Could you check a few things on this model? Use its own coordinates, in mm. A direction names the side the tool comes from. Give positions to 0.01 mm unless a question says otherwise; leave off trailing zeros. Loops run counter-clockwise (first coordinate to the right, second up) from the corner with the lowest first, then second, coordinate; pieces in that order, holes last. Notation, with made-up numbers: (43.5, -21.5) -> (101.5, -21.5) arc R15 cw to (101.5, -3.5) -> close; hole circle Ø5 at (69, 3.5). An arc over 180 degrees is marked (long way). Write each question's results on one line, items separated by ' | '. Start each with the question number.
Q1. Which directions (+Z, -Z, +X, -X, +Y, -Y) give clear straight access to the entire face, cutting with the end or side of a thin tool? Please do faces 5 (the face through (-11.112, 43, 1)), 6 (the face through (30, -30, -50.8)), 7 (the face through (-52.07, 47.74, 0.71)).
Q2. If we section it at D-D, the plane x = 274.5: List the corners of the cut face in (y, z) for me (3 decimals).
Q3. Will these pins go through, and if not, where does the flat tip stop? P1, Ø6, axis at x = 135.5, z = -8, coming from the +Y side; P2, Ø14, axis at y = 44.5, z = -8.5, coming from the +X side; P3, Ø2, axis at x = 180.5, y = -74, coming from the -Z side (3 decimals).
Q4. If we section it at C-C, the plane z = -23.5: List the corners of the cut face in (x, y) for me.
Q5. If I drill on line 1 along Z through (x, y) = (100, -20) (3 decimals); line 2 along X through (y, z) = (8, -6); line 3 along X through (y, z) = (-16, 14), over which ranges is the centre line in solid material (lowest first)?
Q6. If we section it at B-B, the plane x = 0: List the corners of the cut face in (y, z) for me (3 decimals), plus the area to 3 significant figures.
Q7. If we section it at A-A, the plane y = 0: List the corners of the cut face in (x, z) for me (3 decimals).
Q8. We'd pull the mould along Y, two halves only. Please class faces 1 (the face through (136.315, 49.845, 0.222)), 2 (the face through (1.519, -38.095, 0.711)), 3 (the face through (172.854, -100.986, 0.222)), 4 (the face through (30, -30, 50.8)): released by +Y, released by -Y, zero draft, split by the parting line, or undercut.
from build123d import *

# Parameters (mm, degrees)
F1_DEPTH = 15.875
F2_R     = 70.64375
F3_DEPTH = 50.8


with BuildPart() as f1:
    # F0 (on Top) → F1 (new body, symmetric)
    with BuildSketch(Plane.XY):
        with BuildLine():
            ThreePointArc((214.0429582689, 78.5021666116), (135.1426887504, 49.6734632535), (51.3239932557, 55.2208007216))
            ThreePointArc((51.3239932557, 55.2208007216), (48.3240107377, 53.8275326792), (49.2448874204, 50.6505723267))
            ThreePointArc((49.2448874204, 50.6505723267), (63.1490502428, -31.6660207082), (-11.1351814225, -69.7606418315))
            ThreePointArc((-11.1351814225, -69.7606418315), (-12.6279755061, -70.6394230316), (-11.8555099032, -72.1899027849))
            ThreePointArc((-11.8555099032, -72.1899027849), (175.5219606246, -100.6779781173), (350.9193591325, -28.8612704918))
            ThreePointArc((350.9193591325, -28.8612704918), (368.6661659856, -22.2694269513), (387.009926427, -26.9500260171))
            ThreePointArc((387.009926427, -26.9500260171), (403.281578789, -31.6726186916), (419.6651697435, -27.3543436198))
            Line((419.6651697435, -27.3543436198), (452.4721534977, -8.2287874757))
            ThreePointArc((452.4721534977, -8.2287874757), (457.1999861821, -0.0162243816), (452.5001585836, 8.212397314))
            Line((452.5001585836, 8.212397314), (419.75852003, 27.4496056792))
            ThreePointArc((419.75852003, 27.4496056792), (401.084074029, 31.7190844567), (383.352674206, 24.4691987482))
            ThreePointArc((383.352674206, 24.4691987482), (338.4707971933, 14.2282569652), (303.7446396069, 44.45))
            Line((303.7446396069, 44.45), (214.0429582689, 78.5021666116))
        make_face()
    extrude(amount=F1_DEPTH, both=True)

    # F2 (on Top) → F3 (join, symmetric)
    with BuildSketch(Plane.XY):
        Circle(F2_R)
        with BuildLine():
            ThreePointArc((11.1125, 36.46996667), (0, -38.1254), (-11.1125, 36.46996667))
            Line((-11.1125, 36.46996667), (-11.1125, 49.1236))
            Line((-11.1125, 49.1236), (11.1125, 49.1236))
            Line((11.1125, 49.1236), (11.1125, 36.46996667))
        make_face(mode=Mode.SUBTRACT)
    extrude(amount=F3_DEPTH, both=True)


solid = f1.part
Final values:
1) face 5: +Z, -Z | face 6: -Z, +X, -X, +Y, -Y | face 7: none
2) outline: (-73.974, -15.875) -> (55.552, -15.875) -> (55.552, 15.875) -> (-73.974, 15.875) -> close
3) P1: stops at y = 50.18 | P2: stops at x = 307.2 | P3: stops at z = -15.875
4) outline: circle Ø141.29 at (0, 0); hole (-11.11, 36.47) arc R38.13 ccw (long way) to (11.11, 36.47) -> (11.11, 49.12) -> (-11.11, 49.12) -> close
5) line 1: z = -15.875 to 15.875 | line 2: x = -70.19 to -37.28, 37.28 to 452.84 | line 3: x = -68.81 to -34.61, 34.61 to 439.14
6) outline: (-77.238, -15.875) -> (-70.644, -15.875) -> (-70.644, -50.8) -> (-38.125, -50.8) -> (-38.125, 50.8) -> (-70.644, 50.8) -> (-70.644, 15.875) -> (-77.238, 15.875) -> close; (49.124, -50.8) -> (70.644, -50.8) -> (70.644, 50.8) -> (49.124, 50.8) -> close | area: 5,700 mm²
7) outline: (-70.644, -50.8) -> (-38.125, -50.8) -> (-38.125, 50.8) -> (-70.644, 50.8) -> close; (38.125, -50.8) -> (70.644, -50.8) -> (70.644, -15.875) -> (457.2, -15.875) -> (457.2, 15.875) -> (70.644, 15.875) -> (70.644, 50.8) -> (38.125, 50.8) -> close
8) face 1: released by +Y | face 2: undercut | face 3: released by -Y | face 4: zero draft
